Model file for the job. Use its own axes, mm. A direction names the side the tool comes from. Coordinates: 2 decimals unless noted, no trailing zeros. Write each loop counter-clockwise with the first axis right and the second up, starting at its lowest first coordinate (ties: lowest second). Pieces come first, ordered by that corner, then holes.
Q1. Band-saw the part on C-C, the plane y = 5.75. Write the cut outline in (x, z), plus the area to 3 significant figures.
Q2. Band-saw the part on B-B, the plane z = 8. Write the cut outline in (x, y) (3 decimals).
Q3. Pull direction Y, two halves, no side cores. Call faces 1 (the flat face through (-4, 12, -3.55)), 2 (the cylindrical face through (-7.05, 7.613, 8.843)), 3 (the cylindrical face through (-1.1, 9.58, 16.87)), 4 (the flat face through (-7, 0, 5)): released by +Y, released by -Y, zero draft, split by the parting line, or undercut.
Q4. Band-saw the part on D-D, the plane x = -2.25. Write the cut outline in (y, z) (3 decimals).
Q5. Pin check, flat tips, straight feed: P1, Ø1, axis at y = 12.5, z = -1.5, coming from the -X side; P2, Ø1, axis at x = -5, z = 13, coming from the +Y side; P3, Ø4, axis at x = -3, z = -2.5, coming from the -Y side. Stop position of each tip, or through.
Q6. Band-saw the part on A-A, the plane x = -7.15. Write the cut outline in (y, z) (3 decimals), plus the area to 3 significant figures.
Q7. Which spindle directions (+Z, -Z, +X, -X, +Y, -Y) get a long thin tool onto all of the face, cutting with end or side? Do faces 5 (the flat face through (0, 7, 5)), 6 (the cylindrical face through (-11.683, 2.919, 12.599)), 7 (the flat face through (-8.35, 12, -2)), 8 (the flat face through (-4, 10.7, -2)), 9 (the flat face through (-7, 7, 19.3)). Say none if no direction does.
Q8. Drill centre lines: probe 1 along Y at (x, z) = (-6, 8) (3 decimals); probe 2 along Z at (x, y) = (-1, 5.5); probe 3 along Z at (x, y) = (-9.5, 7). Where is each one in solid material? Low to high.
Autodesk Inventor part; units mm, degrees
ref_plane "Work Plane1" through (0, 7.075, 10.75) normal (0, 0, 1) x (1, 0, 0)
ref_plane "YZ Plane" through (0, 0, 0) normal (1, 0, 0) x (0, 1, 0)
ref_plane "XZ Plane" through (0, 0, 0) normal (0, 1, 0) x (-1, 0, 0)
sketch "Sketch1" plane through (0, 0, 0) normal (0, 0, 1) x (1, 0, 0)
  line L0 (0, 0) -> (-14.3, 0)
  line L1 (-14.3, 0) -> (-14.3, 14.15)
  line L2 (-14.3, 14.15) -> (0, 14.15)
  line L3 (0, 14.15) -> (0, 0)
  dimension "d0" = 14.15
  dimension "d1" = 14.3
extrude "Extrusion1" add sketch "Sketch1" along normal blind 8
sketch "Sketch2" plane through (0, 0, 0) normal (1, 0, 0) x (0, 0, -1)
  line L0 (0, 0) -> (0, 14.15)
  line L1 (0, 14.15) -> (-8, 14.15)
  line L2 (-8, 0) -> (-8, 14.15)
  line L3 (0, 0) -> (-8, 0)
  line L4 (0, 0) -> (0, 14.15) construction
  line L5 (0, 7.075) -> (-10.75, 7.075) construction
  line L6 (-8, 0) -> (-8, 14.15)
  circle A0 centre (-8, 7.075) radius 1
  circle A1 centre (-8, 7.075) radius 2.75
  point P0 (-8, 9.825)
  point P1 (-8, 4.325)
  point P2 (-8, 8.075)
  point P3 (-8, 6.075)
  dimension "d4" = 10.75
  dimension "d5" = 2
extrude "Extrusion2" add sketch "Sketch2" against normal up to surface (14.3 mm away) contours A1 L2 A0 | A0 L2 picked at (-9.5833, 8.5314) picked at (-8.3098, 7.4083)
extrude "Extrusion3" cut sketch "Sketch2" against normal up to surface (14.3 mm away) contours A0 L2 | L2 A0
ref_plane "Work Plane1" through (0, 7.075, 10.75) normal (0, 0, 1) x (1, 0, 0)
sketch "Sketch3" plane through (0, 7.075, 10.75) normal (0, 0, 1) x (1, 0, 0)
  line L0 (-14.3, 2.75) -> (0, 2.75)
  line L1 (0, 2.75) -> (0, 7.075)
  line L2 (0, 7.075) -> (-14.3, 7.075)
  line L3 (-14.3, 7.075) -> (-14.3, 2.75)
  line L4 (0, -2.75) -> (-14.3, -2.75)
  line L5 (-14.3, -2.75) -> (-14.3, -7.075)
  line L6 (-14.3, -7.075) -> (0, -7.075)
  line L7 (0, -7.075) -> (0, -2.75)
  line L8 (-14.3, 2.75) -> (-14.3, -2.75)
  line L9 (0, -2.75) -> (-14.3, -2.75)
  line L10 (0, 2.75) -> (0, -2.75)
  line L11 (-14.3, 2.75) -> (0, 2.75)
  line L12 (0, 7.075) -> (-14.3, 7.075) construction
  line L13 (-7.15, 7.075) -> (-7.15, -7.075) construction
  line L14 (-14.3, -7.075) -> (0, -7.075) construction
  circle A0 centre (-7.15, 0) radius 6.15
  dimension "d10" = 12.3
extrude "Extrusion4" add sketch "Sketch3" against normal up to surface (2.75 mm away) contours A0 L0 | L0 A0 L4 | L4 A0
extrude "Extrusion5" cut sketch "Sketch2" against normal up to surface (14.3 mm away) contours A0 L2 picked at (-8.3098, 7.4083)
extrude "Extrusion6" add sketch "Sketch3" along normal blind 8 contours A0 L0 | L0 A0 L4 | L4 A0
sketch "Sketch4" plane through (0, 0, 0) normal (1, 0, 0) x (0, 0, -1)
  line L0 (0, 0) -> (0, 14.15) construction
  line L1 (0, 7.075) -> (-14.5, 7.075) construction
  line L2 (-18.75, 0.925) -> (-8, 0.925) construction
  line L3 (-14.5, 0.925) -> (-23.2095, 0.925)
  line L4 (-23.2095, 0.925) -> (-23.2095, 17.6688)
  line L5 (-23.2095, 17.6688) -> (-14.5, 17.6688)
  line L6 (-14.5, 17.6688) -> (-14.5, 0.925)
  dimension "d17" = 14.5
extrude "Extrusion7" cut sketch "Sketch4" against normal through all
sketch "Sketch5" plane through (-7.15, 7.075, 14.5) normal (0, 0, 1) x (1, 0, 0)
  circle A0 centre (0, 0) radius 6.55
  point P0 (7.15, -7.075)
  dimension "d20" = 13.1
extrude "Extrusion8" add sketch "Sketch5" along normal blind 8
sketch "Sketch6" plane through (0, 0, 0) normal (1, 0, 0) x (0, 0, -1)
  circle A0 centre (-8, 7.075) radius 1 construction
  line L0 (0, 0) -> (0, 14.15) construction
  line L1 (0, 14.15) -> (-8, 14.15) construction
  line L2 (-8, 9.825) -> (-8, 14.15) construction
  arc A1 (-8, 9.825) -> (-8, 4.325) centre (-8, 7.075) ccw construction
  line L3 (-8, 0) -> (-8, 4.325) construction
  line L4 (0, 0) -> (-8, 0) construction
  line L5 (0, 14.15) -> (0, 0) construction
  line L6 (0, 7.075) -> (-19.3, 7.075) construction
  line L7 (-14.5, 0.525) -> (-22.5, 0.525)
  line L8 (-19.3, 0.525) -> (-27.8316, 0.525)
  line L9 (-27.8316, 0.525) -> (-27.8316, 15.7859)
  line L10 (-27.8316, 15.7859) -> (-19.3, 15.7859)
  line L11 (-19.3, 15.7859) -> (-19.3, 0.525)
  dimension "d23" = 19.3
extrude "Extrusion9" cut sketch "Sketch6" against normal through all
fillet "Fillet1" radius 5 4 edges at (-0.8245, 4.325, 8) (-0.8245, 9.825, 8) (-13.4755, 4.325, 8) (-13.4755, 9.825, 8)
sketch "Sketch7" plane through (0, 0, 0) normal (0, 0, -1) x (-1, 0, 0)
  line L0 (14.3, 0) -> (0, 0)
  line L1 (14.3, 14.15) -> (14.3, 0)
  line L2 (0, 14.15) -> (14.3, 14.15)
  line L3 (0, 0) -> (0, 14.15)
  line L4 (0, 14.15) -> (14.3, 14.15)
  line L5 (0, 14.15) -> (8.35, 14.15)
  line L6 (8.35, 14.15) -> (8.35, 10.7)
  line L7 (8.35, 10.7) -> (0, 10.7)
  line L8 (0, 10.7) -> (0, 14.15)
  dimension "d28" = 8.35
  dimension "d29" = 3.45
extrude "Extrusion10" add sketch "Sketch7" along normal blind 3.55 contours L3 L2 L6 L7
sketch "Sketch8" plane through (0, 7.075, 10.75) normal (0, 0, 1) x (1, 0, 0)
  line L0 (0, 7.075) -> (-14.3, 7.075)
  line L1 (-14.3, -7.075) -> (0, -7.075)
  line L2 (-14.3, 7.075) -> (-14.3, -7.075)
  line L3 (0, -7.075) -> (0, 7.075)
extrude "Extrusion11" add sketch "Sketch8" against normal up to surface (2.75 mm away)
extrude "Extrusion12" cut sketch "Sketch2" against normal up to surface (14.3 mm away) contours A0 L2 picked at (-8.3098, 7.4083)
sketch "Sketch9" plane through (0, 0, 0) normal (1, 0, 0) x (0, 0, -1)
  circle A0 centre (-8, 7.075) radius 1
  line L0 (0, 0) -> (-10.75, 0)
  line L1 (0, 0) -> (0, 10.7)
  line L2 (0, 10.7) -> (3.55, 10.7)
  line L3 (3.55, 14.15) -> (3.55, 10.7)
  line L4 (3.55, 14.15) -> (-10.75, 14.15)
  line L5 (-10.75, 0) -> (-10.75, 14.15)
  line L6 (0, 7.075) -> (-142.5994, 7.075)
  line L7 (0, 7.075) -> (195.5312, 7.075)
properties part number "dummy camera"
Answer sheet:
1. outline: (-14.3, 0) - (0, 0) - (0, 10.75) - (-1.14, 10.75) - (-1.14, 14.5) - (-0.74, 14.5) - (-0.74, 19.3) - (-13.56, 19.3) - (-13.56, 14.5) - (-13.16, 14.5) - (-13.16, 10.75) - (-14.3, 10.75) - close
1. area: 260 mm2
2. outline: (-14.3, 0) - (0, 0) - (0, 6.075) - (-14.3, 6.075) - close; (-14.3, 8.075) - (0, 8.075) - (0, 14.15) - (-14.3, 14.15) - close
3. face 1: zero draft
3. face 2: undercut
3. face 3: split by the parting line
3. face 4: released by -Y
4. outline: (0, 0) - (10.7, 0) - (10.7, -3.55) - (14.15, -3.55) - (14.15, 10.75) - (10.792, 10.75) - (10.792, 14.5) - (11.422, 14.5) - (11.422, 19.3) - (2.728, 19.3) - (2.728, 14.5) - (3.358, 14.5) - (3.358, 10.75) - (0, 10.75) - close; hole circle Ø2 at (7.075, 8)
5. P1: stops at x = -8.35
5. P2: stops at y = 13
5. P3: stops at y = 10.7
6. outline: (0, 0) - (10.7, 0) - (10.7, -3.55) - (14.15, -3.55) - (14.15, 10.75) - (13.225, 10.75) - (13.225, 14.5) - (13.625, 14.5) - (13.625, 19.3) - (0.525, 19.3) - (0.525, 14.5) - (0.925, 14.5) - (0.925, 10.75) - (0, 10.75) - close; hole circle Ø2 at (7.075, 8)
6. area: 270 mm2
7. face 5: +Z, -Z, +X, +Y, -Y
7. face 6: none
7. face 7: -Z, -X, +Y, -Y
7. face 8: -Z, +X, -X, -Y
7. face 9: +Z, +X, -X, +Y, -Y
8. probe 1: y = 0 to 6.075, 8.075 to 14.15
8. probe 2: z = 0 to 10.75, 14.5 to 19.3
8. probe 3: z = 0 to 7, 9 to 19.3
